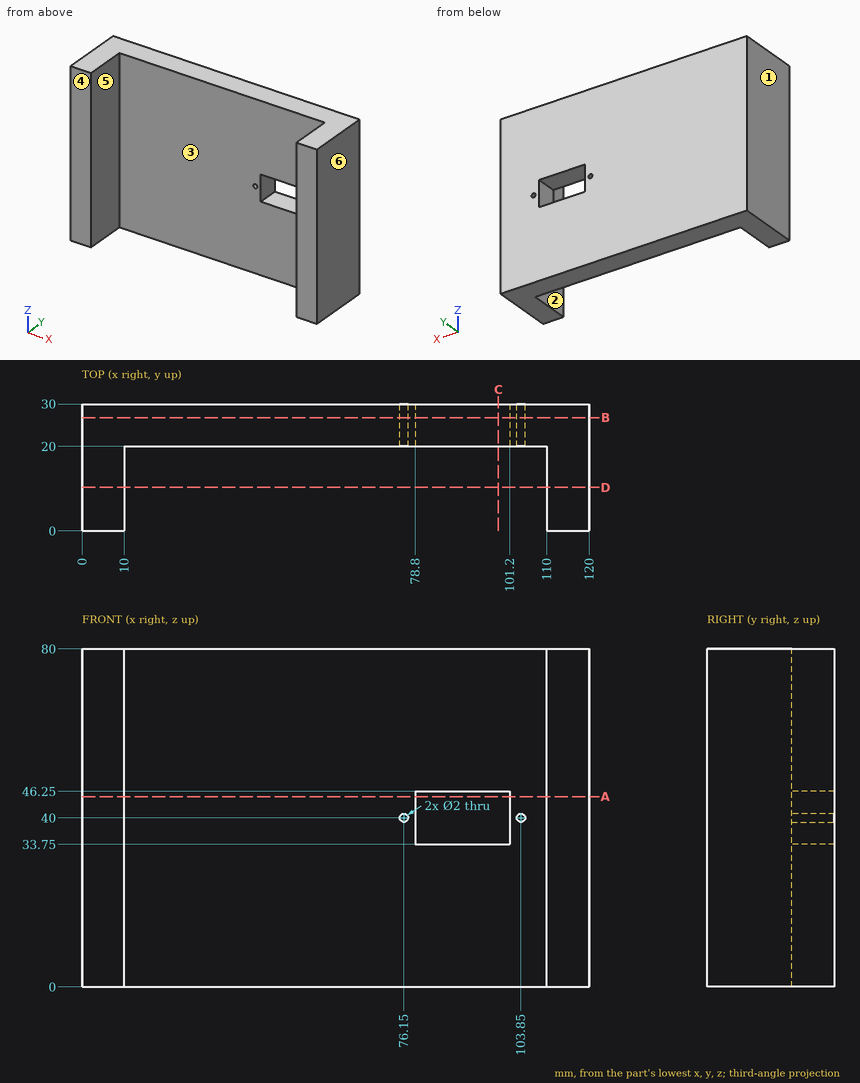
Answer from the drawing. Dimensions are ordinates in mm from the lowest x, y and z of the part. A direction names the side the tool comes from. Coordinates: 2 decimals unless noted, no trailing zeros. Loops run counter-clockwise (first coordinate to the right, second up) from the corner with the lowest first, then second, coordinate; pieces in that order, holes last.
Q1. The part is cut by section D-D on y = 10.25. Write down the section's boundary in (x, z), and give its area (3 significant figures).
Q2. The part is cut by section A-A on z = 45. Write down the section's boundary in (x, y).
Q3. This flat-tipped pin is pushed along its axis until it touches: pin 1 Ø5 at (x, z) = (57, 21) entering from -Y. Where does it stop, or does it pass through?
Q4. Consider probe 1 along X at (y, z) = (26.75, 40); probe 2 along Z at (x, y) = (103.85, 23); probe 3 along X at (y, z) = (21.25, 41.5). Determine where each line is inside the solid, lowest interval first.
Q5. The mould has two halves that part along X. Classify the marked faces 1, 2, 3 and 4: +X half, -X half, draft (parallel to the pull), parting line (faces both ways), or undercut.
Q6. The part is cut by section B-B on y = 26.75. Write down the section's boundary in (x, z).
Q7. The part is cut by section C-C on x = 98.5. Write down the section's boundary in (y, z).
Q8. Which of the six approach directions +Z, -Z, +X, -X, +Y, -Y give full straight-line access (tool end or side, diameter ignored) to the marked faces 5 and 6?
Results below:
1. outline: (0, 0) - (10, 0) - (10, 80) - (0, 80) - close; (110, 0) - (120, 0) - (120, 80) - (110, 80) - close
1. area: 1,600 mm2
2. outline: (0, 0) - (10, 0) - (10, 20) - (78.8, 20) - (78.8, 30) - (0, 30) - close; (101.2, 20) - (110, 20) - (110, 0) - (120, 0) - (120, 30) - (101.2, 30) - close
3. pin 1: stops at y = 20
4. probe 1: x = 0 to 75.15, 77.15 to 78.8, 101.2 to 102.85, 104.85 to 120
4. probe 2: z = 0 to 39, 41 to 80
4. probe 3: x = 0 to 78.8, 101.2 to 120
5. face 1: -X half
5. face 2: undercut
5. face 3: undercut
5. face 4: draft
6. outline: (0, 0) - (120, 0) - (120, 80) - (0, 80) - close; hole circle Ø2 at (76.15, 40); hole (78.8, 33.75) - (101.2, 33.75) - (101.2, 46.25) - (78.8, 46.25) - close; hole circle Ø2 at (103.85, 40)
7. outline: (20, 0) - (30, 0) - (30, 33.75) - (20, 33.75) - close; (20, 46.25) - (30, 46.25) - (30, 80) - (20, 80) - close
8. face 5: +Z, -Z, -Y
8. face 6: +Z, -Z, +X, +Y, -Y
